Part model, mm, in its own coordinate system. A direction names the side the tool comes from. Give positions to 0.01 mm unless a question says otherwise; leave off trailing zeros. Write each loop counter-clockwise with the first axis right and the second up, starting at its lowest first coordinate (ties: lowest second). Pieces come first, ordered by that corner, then holes. Notation, with made-up numbers: M 15.25,65.25 L 51.25,65.25 A24 cw 51.25,93.25 Z; hole C -8.75,75.5 d3. An arc over 180 degrees is marked long. Use CSV: the item, a comma, the result in double quotes. Start each with the question number.
1. Band-saw the part on D-D, the plane x = -16. List the corners of the cut face in (y, z).
2. Band-saw the part on B-B, the plane y = 61.5. List the corners of the cut face in (x, z).
3. 3-axis set-ups, long thin cutter, end or side, ignore diameter. For faces 4 (the face through (87.814, 48, 18)), 5 (the face through (-53.8, 49, -1)), 6 (the face through (-68.514, 48, -1)), 7 (the face through (-66.514, 48, 0)), 8 (the face through (-61, 24.3, -1)): which of +Z, -Z, +X, -X, +Y, -Y reach the whole face in a straight line?
4. Band-saw the part on A-A, the plane x = -39. List the corners of the cut face in (y, z), then the cut area to 3 significant figures.
5. Mould opens along X. For faces 1 (the face through (-70.388, 95.496, 16.269)), 2 (the face through (-34.036, 48, 1)), 3 (the face through (10, 0, 17)) say: pulls with the +X half, pulls with the -X half, needs draft (parallel to the pull), parting line crosses it, or undercut.
6. Band-saw the part on C-C, the plane z = 24. List the corners of the cut face in (x, y).
7. Drop flat-ended pins along their axis: pin 1 Ø4 at (x, y) = (44.5, 82.5) entering from +Z; pin 2 Ø3.5 at (x, z) = (-60, -2) entering from +Y; pin 3 Ø0.9 at (y, z) = (59.5, -1) entering from -X. Give the stop position or say it passes through.
8. Drill centre lines: line 1 along X through (y, z) = (40.5, 1); line 2 along X through (y, z) = (59, 20); line 3 along Y through (x, z) = (33.5, 6.5). Where is each one in solid material? Low to high. Write a range as from..to.
from build123d import *

# Parameters (mm, degrees)
CROQUIS1_W                = 10.714275766
CROQUIS1_H                = 44.4
SALIENTE_EXTRUIR1_DEPTH   = 3
SALIENTE_EXTRUIR1_2_DEPTH = 3
CROQUIS2_W                = 143.628551532
CROQUIS2_H                = 97
CROQUIS2_W_2              = 17.964463827
CROQUIS2_H_2              = 35
CROQUIS2_W_3              = 10.714275766
CROQUIS2_H_3              = 44.4
SALIENTE_EXTRUIR2_DEPTH   = 3
CROQUIS3_W                = 143.628551532
CROQUIS3_H                = 97
CROQUIS3_W_2              = 137.628551532
CROQUIS3_H_2              = 91
SALIENTE_EXTRUIR3_DEPTH   = 30
REDONDEO1_R               = 5
CROQUIS4_W                = 35.073435796
CROQUIS4_H                = 97.224073942
CORTAR_EXTRUIR1_DEPTH     = 5
CORTAR_EXTRUIR2_START     = -3
CROQUIS6_W                = 10.714275766
CROQUIS6_H                = 44.4
CORTAR_EXTRUIR2_DEPTH     = 3
CROQUIS7_W                = 3
CROQUIS7_H                = 44.4
SALIENTE_EXTRUIR4_DEPTH   = 11
SALIENTE_EXTRUIR5_DEPTH   = 26
CROQUIS9_W                = 5
CROQUIS9_H                = 91
SALIENTE_EXTRUIR6_DEPTH   = 30
REDONDEO2_R               = 3


with BuildPart() as part:
    # Croquis1 → Saliente-Extruir1 (new body)
    with BuildSketch(Plane.XY):
        with BuildLine():
            ThreePointArc((-54.8, 72.7), (-54.092893219, 72.407106781), (-53.8, 71.7))
            Line((-53.8, 71.7), (-53.8, 25.3))
            ThreePointArc((-53.8, 25.3), (-54.092893219, 24.592893219), (-54.8, 24.3))
            Line((-54.8, 24.3), (-67.514275766, 24.3))
            ThreePointArc((-67.514275766, 24.3), (-68.221382548, 24.592893219), (-68.514275766, 25.3))
            Line((-68.514275766, 25.3), (-68.514275766, 71.7))
            ThreePointArc((-68.514275766, 71.7), (-68.221382548, 72.407106781), (-67.514275766, 72.7))
            Line((-67.514275766, 72.7), (-54.8, 72.7))
        make_face()
        with Locations((-61.157137883, 48.5)):
            Rectangle(CROQUIS1_W, CROQUIS1_H, mode=Mode.SUBTRACT)
    extrude(amount=-SALIENTE_EXTRUIR1_DEPTH)



with BuildPart() as body_2:
    # Croquis1 → Saliente-Extruir1 2 (new body)
    with BuildSketch(Plane.XY):
        with BuildLine():
            ThreePointArc((68.514275766, 25.3), (68.221382548, 24.592893219), (67.514275766, 24.3))
            Line((67.514275766, 24.3), (54.8, 24.3))
            ThreePointArc((54.8, 24.3), (54.092893219, 24.592893219), (53.8, 25.3))
            Line((53.8, 25.3), (53.8, 71.7))
            ThreePointArc((53.8, 71.7), (54.092893219, 72.407106781), (54.8, 72.7))
            Line((54.8, 72.7), (67.514275766, 72.7))
            ThreePointArc((67.514275766, 72.7), (68.221382548, 72.407106781), (68.514275766, 71.7))
            Line((68.514275766, 71.7), (68.514275766, 25.3))
        make_face()
        with Locations((61.157137883, 48.5)):
            Rectangle(CROQUIS1_W, CROQUIS1_H, mode=Mode.SUBTRACT)
    extrude(amount=-SALIENTE_EXTRUIR1_2_DEPTH)


with BuildPart() as part_1:
    add(part.part)

    add(body_2.part)  # Saliente-Extruir2 merges body 2
    # Croquis2 → Saliente-Extruir2 (add)
    with BuildSketch(Plane.XY):
        with Locations((0, 48.5)):
            Rectangle(CROQUIS2_W, CROQUIS2_H)
        with Locations((-43.017768086, 48.5)):
            Rectangle(CROQUIS2_W_2, CROQUIS2_H_2, mode=Mode.SUBTRACT)
        with Locations((61.157137883, 48.5)):
            Rectangle(CROQUIS2_W_3, CROQUIS2_H_3, mode=Mode.SUBTRACT)
        with Locations((-61.157137883, 48.5)):
            Rectangle(CROQUIS2_W_3, CROQUIS2_H_3, mode=Mode.SUBTRACT)
    extrude(amount=SALIENTE_EXTRUIR2_DEPTH)

    # Croquis3 → Saliente-Extruir3 (add)
    with BuildSketch(Plane.XY.offset(3)):
        with Locations((0, 48.5)):
            Rectangle(CROQUIS3_W, CROQUIS3_H)
        with Locations((0, 48.5)):
            Rectangle(CROQUIS3_W_2, CROQUIS3_H_2, mode=Mode.SUBTRACT)
    extrude(amount=SALIENTE_EXTRUIR3_DEPTH)

    # Redondeo1
    redondeo1_edges = [part_1.edges().sort_by_distance(p)[0] for p in [
        (71.814275766, 0, 16.5),
        (71.814275766, 97, 16.5),
        (-71.814275766, 97, 16.5),
        (-71.814275766, 0, 16.5),
    ]]
    fillet(redondeo1_edges, radius=REDONDEO1_R)

    # Croquis4 → Cortar-Extruir1 (cut)
    with BuildSketch(Plane(origin=(71.814275766, 0, 0), x_dir=(0, 0, -1), z_dir=(1, 0, 0))):
        with Locations((-17.536717898, 48.612036971)):
            Rectangle(CROQUIS4_W, CROQUIS4_H)
    extrude(amount=-CORTAR_EXTRUIR1_DEPTH, mode=Mode.SUBTRACT)

    # Croquis6 → Cortar-Extruir2 (cut)
    with BuildSketch(Plane(origin=(0, 0, -3), x_dir=(-1, 0, 0), z_dir=(0, 0, -1)).offset(CORTAR_EXTRUIR2_START)):
        with BuildLine():
            Line((-67.514275766, 24.3), (-54.8, 24.3))
            ThreePointArc((-54.8, 24.3), (-54.092893219, 24.592893219), (-53.8, 25.3))
            Line((-53.8, 25.3), (-53.8, 71.7))
            ThreePointArc((-53.8, 71.7), (-54.092893219, 72.407106781), (-54.8, 72.7))
            Line((-54.8, 72.7), (-67.514275766, 72.7))
            ThreePointArc((-67.514275766, 72.7), (-68.221382548, 72.407106781), (-68.514275766, 71.7))
            Line((-68.514275766, 71.7), (-68.514275766, 25.3))
            ThreePointArc((-68.514275766, 25.3), (-68.221382548, 24.592893219), (-67.514275766, 24.3))
        make_face()
        with Locations((-61.157137883, 48.5)):
            Rectangle(CROQUIS6_W, CROQUIS6_H, mode=Mode.SUBTRACT)
    extrude(amount=CORTAR_EXTRUIR2_DEPTH, mode=Mode.SUBTRACT)

    # Croquis7 → Saliente-Extruir4 (add)
    with BuildSketch(Plane(origin=(55.8, 0, 0), x_dir=(0, 0, -1), z_dir=(1, 0, 0))):
        with Locations((-1.5, 48.5)):
            Rectangle(CROQUIS7_W, CROQUIS7_H)
    extrude(amount=SALIENTE_EXTRUIR4_DEPTH)

    # Croquis8 → Saliente-Extruir5 (add)
    with BuildSketch(Plane(origin=(66.814275766, 0, 0), x_dir=(0, 0, -1), z_dir=(1, 0, 0))):
        Polygon((-33, 0), (0, 0), (0, 97), (-33, 97), (-33, 94), (-3, 94), (-3, 3), (-33, 3), align=None)
    extrude(amount=SALIENTE_EXTRUIR5_DEPTH)

    # Croquis9 → Saliente-Extruir6 (add)
    with BuildSketch(Plane.XY.offset(3)):
        with Locations((90.314275766, 48.5)):
            Rectangle(CROQUIS9_W, CROQUIS9_H)
    extrude(amount=SALIENTE_EXTRUIR6_DEPTH)

    # Redondeo2
    redondeo2_edges = [part_1.edges().sort_by_distance(p)[0] for p in [
        (92.814275766, 0, 16.5),
        (92.814275766, 97, 16.5),
    ]]
    fillet(redondeo2_edges, radius=REDONDEO2_R)


solid = part_1.part
Output:
1,outline,"M 0,0 L 97,0 L 97,33 L 94,33 L 94,3 L 3,3 L 3,33 L 0,33 Z"
2,outline,"M -71.81,0 L -68.51,0 L -68.51,-3 L -66.51,-3 L -66.51,3 L -68.81,3 L -68.81,33 L -71.81,33 Z; M -55.8,-3 L -53.8,-3 L -53.8,0 L -52,0 L -52,3 L -55.8,3 Z; M -34.04,0 L 92.81,0 L 92.81,33 L 87.81,33 L 87.81,3 L -34.04,3 Z"
3,face 4,"+Z"
3,face 5,"-Z, +X, +Y, -Y"
3,face 6,"-Z, -X, +Y, -Y"
3,face 7,"+Z, -Z"
3,face 8,"-Z, +X, -X, -Y"
4,outline,"M 0,0 L 31,0 L 31,3 L 3,3 L 3,33 L 0,33 Z; M 66,0 L 97,0 L 97,33 L 94,33 L 94,3 L 66,3 Z"
4,area,"366 mm²"
5,face 1,"pulls with the -X half"
5,face 2,"undercut"
5,face 3,"needs draft"
6,outline,"M -71.81,5 A5 ccw -66.81,0 L 89.81,0 A3 ccw 92.81,3 L 92.81,94 A3 ccw 89.81,97 L -66.81,97 A5 ccw -71.81,92 Z; hole M -68.81,3 L 87.81,3 L 87.81,94 L -68.81,94 Z"
7,pin 1,"stops at z = 3"
7,pin 2,"stops at y = 72.7"
7,pin 3,"stops at x = -68.51"
8,line 1,"x = -71.81..-66.51, -55.8..-52, -34.04..92.81"
8,line 2,"x = -71.81..-68.81, 87.81..92.81"
8,line 3,"y = 0..3, 94..97"
